Design review of the part built by this model. Coordinates are the model's own, in mm. A direction names the side the tool comes from. Coordinates: 2 decimals unless noted, no trailing zeros. Loops run counter-clockwise (first coordinate to the right, second up) from the corner with the lowest first, then second, coordinate; pieces in that order, holes last. Notation, with made-up numbers: (77, 55) - (93, 55) arc R25 cw to (93, 83) - close; hole circle Ø2 at (43, 3). An arc over 180 degrees is marked (long way). Answer in a Markdown table with one row per item. Add a question column.
(1) To check wall thickness, follow L1, parallel to Y at x = 0, z = 0.6; L2, parallel to Z at x = 1.25, y = 3.25; L3, parallel to Y at x = -3.75, z = 1.1. State the ranges of each line that lie inside material, in increasing order. Write a range as [from, to].
(2) The part is to be moulded in two halves that separate along Y. For faces 1 (the face through (0, 0, 4)), 2 (the face through (4.25, -2.02, 2.52)), 3 (the face through (-4.25, -2.02, 2.52)), 4 (the face through (0, 4.5, 2)), say which applies: released by +Y, released by -Y, zero draft, split by the parting line, or undercut.
(3) For faces 5 (the face through (-4.847, -0.063, 1.747)), 6 (the face through (0, -11, 2)), 7 (the face through (4.847, -0.063, 1.747)), 8 (the face through (-1, 6, 1)), list the 3-axis set-ups (+Z, -Z, +X, -X, +Y, -Y) from which the entire face can be reached by the end or side of a thin tool; tool diameter is ignored.
(4) We need section C-C, the plane y = 8. Write out the cut boundary in (x, z).
(5) We need section A-A, the plane y = -11.25. Write out the cut boundary in (x, z) (3 decimals), plus the area to 3 significant figures.
(6) Clearance check with flat-ended pins moving along their axes: pin 1 (1 mm diameter, centred on x = -3, z = 3, fed in from -Y); pin 2 (0.8 mm diameter, centred on x = -1, z = 2, fed in from +Y); pin 3 (1 mm diameter, centred on y = 3.5, z = 1.5, fed in from -X); pin 4 (2 mm diameter, centred on x = 1.5, z = 2.5, fed in from -Y). State where each tip first meets the part, or that it passes through.
from build123d import *

# Parameters (mm, degrees)
SKETCH2_W                = 10
SKETCH2_H                = 9
BOSS_EXTRUDE1_DEPTH      = 4
CHAMFER1_SIZE            = 0.5
CUT_EXTRUDE1_DEPTH       = 3
BOSS_EXTRUDE2_DEPTH      = 0.4
LPATTERN1_COUNT          = 2
LPATTERN1_PITCH          = 2.54
LPATTERN2_COUNT          = 2
LPATTERN2_PITCH          = 2.54
DRAFT2_ANGLE             = -5
SKETCH8_R                = 1.98
BOSS_EXTRUDE3_DEPTH      = 0.01
BOSS_EXTRUDE3_DEPTH_BACK = 1
FILLET1_R                = 0.5


with BuildPart() as part:
    # Sketch2 → Boss-Extrude1 (new body)
    with BuildSketch(Plane.XY):
        Rectangle(SKETCH2_W, SKETCH2_H)
    extrude(amount=BOSS_EXTRUDE1_DEPTH)

    # Chamfer1
    chamfer1_edges = [part.edges().sort_by_distance(p)[0] for p in [
        (0, 4.5, 4),
    ]]
    chamfer(chamfer1_edges, length=CHAMFER1_SIZE)

    # Sketch6 → Cut-Extrude1 (cut)
    with BuildSketch(Plane.XY.offset(4)):
        with BuildLine():
            Line((5, -1), (5, -3))
            ThreePointArc((5, -3), (4.25, -2), (5, -1))
        make_face()
    cut_extrude1 = extrude(amount=-CUT_EXTRUDE1_DEPTH, mode=Mode.SUBTRACT)

    # Mirror1: Cut-Extrude1 across plane
    add(cut_extrude1.mirror(Plane(origin=(0, 0, 0), x_dir=(0, 0, 1), z_dir=(1, 0, 0))), mode=Mode.SUBTRACT)

    # Sketch7 → Boss-Extrude2 (add)
    with BuildSketch(Plane.XY.offset(2)):
        Polygon((-0.57, -4.5), (-0.57, -8.44), (-0.375, -8.44), (-0.375, -16.44), (-0.25, -17.2), (0.25, -17.2), (0.375, -16.44), (0.375, -8.44), (0.57, -8.44), (0.57, -4.5), align=None)
    boss_extrude2 = extrude(amount=BOSS_EXTRUDE2_DEPTH)

    # LPattern1: Boss-Extrude2 ×2
    with Locations(*[(-i * LPATTERN1_PITCH, 0, 0) for i in range(1, LPATTERN1_COUNT)]):
        add(boss_extrude2)

    # LPattern2: Boss-Extrude2 ×2
    with Locations(*[(i * LPATTERN2_PITCH, 0, 0) for i in range(1, LPATTERN2_COUNT)]):
        add(boss_extrude2)

    # Draft2
    draft2_faces = [part.faces().sort_by_distance(p)[0] for p in [
        (5, 0.383542538, 1.891910739),
        (-5, 0.383542538, 1.891910739),
    ]]
    draft(draft2_faces, Plane(origin=(0, 0, 0), x_dir=(-1, 0, 0), z_dir=(0, 0, -1)), DRAFT2_ANGLE)

    # Sketch8 → Boss-Extrude3 (add, two sides)
    with BuildSketch(Plane(origin=(0, 0, 0), x_dir=(-1, 0, 0), z_dir=(0, 0, -1))) as boss_extrude3_sk:
        Polygon((-5, 9), (-4, 11), (4, 11), (5, 9), (5, 4.5), (-5, 4.5), align=None)
        with Locations((0, 8)):
            Circle(SKETCH8_R, mode=Mode.SUBTRACT)
    extrude(amount=BOSS_EXTRUDE3_DEPTH)
    extrude(boss_extrude3_sk.sketch, amount=-BOSS_EXTRUDE3_DEPTH_BACK)

    # Fillet1
    fillet1_edges = [part.edges().sort_by_distance(p)[0] for p in [
        (-4.650045346, 1.410302183, 4),
        (4.650045346, 1.410302183, 4),
    ]]
    fillet(fillet1_edges, radius=FILLET1_R)


solid = part.part
Responses:
| question | item | result |
|---|---|---|
| 1 | L1 | y = [-4.5, 6.02], [9.98, 11] |
| 1 | L2 | z = [0, 4] |
| 1 | L3 | y = [-4.5, 4.5] |
| 2 | face 1 | zero draft |
| 2 | face 2 | undercut |
| 2 | face 3 | undercut |
| 2 | face 4 | released by +Y |
| 3 | face 5 | +Z, -X, -Y |
| 3 | face 6 | -Z, +X, -X, -Y |
| 3 | face 7 | +Z, +X, -Y |
| 3 | face 8 | +Z, +X, -X, +Y |
| 4 | outline | (-5, -0.01) - (-1.98, -0.01) - (-1.98, 1) - (-5, 1) - close; (1.98, -0.01) - (5, -0.01) - (5, 1) - (1.98, 1) - close |
| 5 | outline | (-2.915, 2) - (-2.165, 2) - (-2.165, 2.4) - (-2.915, 2.4) - close; (-0.375, 2) - (0.375, 2) - (0.375, 2.4) - (-0.375, 2.4) - close; (2.165, 2) - (2.915, 2) - (2.915, 2.4) - (2.165, 2.4) - close |
| 5 | area | 0.900 mm2 |
| 6 | pin 1 | stops at y = -4.5 |
| 6 | pin 2 | stops at y = 4.5 |
| 6 | pin 3 | stops at x = -4.91 |
| 6 | pin 4 | stops at y = -17.2 |
